from build123d import *

# Parameters (mm, degrees)
F1_DEPTH       = 10
F3_D           = 3.3
F3_CSINK_D     = 6
F3_CSINK_ANGLE = 90
F5_D           = 3.3
F5_CSINK_D     = 6
F5_CSINK_ANGLE = 90


with BuildPart() as f1:
    # F0 (on Front) → F1 (new body)
    with BuildSketch(Plane.XZ):
        Polygon((0, 44), (0, 0), (-15.65, -1.5), (-30.9, 0), (-30.9, 42), (-42.9, 42), (-42.9, 35), (-34.9, 35), (-34.9, -4), (-8, -4), (-8, -11), (4, -11), (4, 48), (-42.9, 48), (-42.9, 44), (-30.9, 44), (-15.65, 45.5), align=None)
    extrude(amount=F1_DEPTH)

    # F3 (through all)
    with Locations(Plane(origin=(0, 0, 35), x_dir=(1, 0, 0), z_dir=(0, 0, -1))):
        with Locations((-38.9, 5)):
            CounterSinkHole(F3_D / 2, F3_CSINK_D / 2, counter_sink_angle=F3_CSINK_ANGLE)

    # F5 (through all)
    with Locations(Plane(origin=(-8, 0, 0), x_dir=(0, -1, 0), z_dir=(-1, 0, 0))):
        with Locations((5, -7.5)):
            CounterSinkHole(F5_D / 2, F5_CSINK_D / 2, counter_sink_angle=F5_CSINK_ANGLE)


solid = f1.part
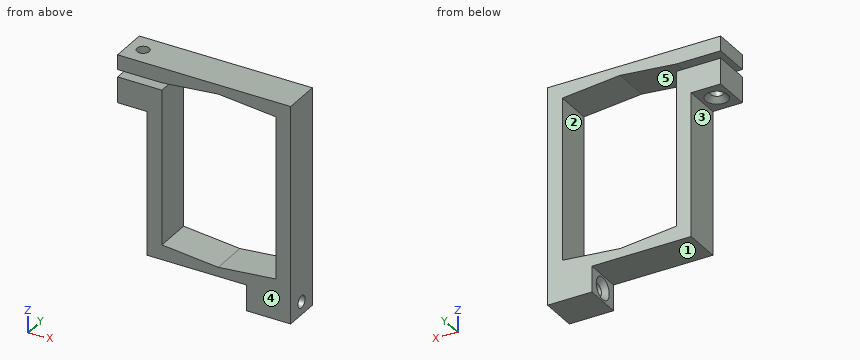
Can you work these out from the model? Positions are in its coordinate system, mm. Face numbers are marked on the shaded views. A direction names the side the tool comes from. Coordinates: 2 decimals unless noted, no trailing zeros. Order: outer loops, then holes, each group sorted by start corner. A loop starts at its lowest first (then second) coordinate and runs counter-clockwise, first axis right, second up. Notation, with made-up numbers: M -7,76 L 12,76 A10 cw 12,94 Z; hole C 7,42 d7. An arc over 180 degrees is marked long. Write item = value, one per line.
(1) Suppose I cut it at A-A on z = 27. Please give me the cut outline in (x, y).
Results are:
outline = M -34.9,-10 L -30.9,-10 L -30.9,0 L -34.9,0 Z; M 0,-10 L 4,-10 L 4,0 L 0,0 Z
(2) Suppose I cut it at C-C on x = -1.5. Please give me the cut outline in (y, z).
Results are:
outline = M -10,-11 L 0,-11 L 0,-0.14 L -10,-0.14 Z; M -10,44.14 L 0,44.14 L 0,48 L -10,48 Z; hole C -5,-7.5 d3.3
(3) Suppose I cut it at B-B on y = -5. State how many separate pieces and enclosed holes the cut face has, plus the area to 3 significant figures.
Results are:
separate_pieces = 4
enclosed_holes = 0
area = 701 mm2
(4) For pin 1 Ø3 at (y, z) = (-3, 28) entering from -X; pin 2 Ø3 at (x, y) = (-16.5, -4.5) entering from -Z; pin 3 Ø5.5 at (y, z) = (-3.5, -7.5) entering from -X; pin 4 Ø2.5 at (x, y) = (-38.9, -5) entering from +Z, each with a flat end and sliding along its axis, tell me the tip position at first contact or that it passes through.
Results are:
pin_1 = -34.9
pin_2 = -4
pin_3 = -8
pin_4 = through
(5) For the marked faces 4 and 5, which set-ups out of +Z, -Z, +X, -X, +Y, -Y let a thin tool reach every point of the face, with its end or its side?
Results are:
face_4 = +Z, -Z, +X, -X, -Y
face_5 = +Y, -Y
(6) Suppose I cut it at D-D on x = -21. Please give me the cut outline in (y, z).
Results are:
outline = M -10,-4 L 0,-4 L 0,-0.97 L -10,-0.97 Z; M -10,44.97 L 0,44.97 L 0,48 L -10,48 Z
(7) If we mould it in two halves opening along Z, with no side actions, what happens to the marked faces 1, 2 and 3? For each: pulls with the +Z half, pulls with the -Z half, needs draft (parallel to the pull), parting line crosses it, or undercut.
Results are:
face_1 = pulls with the -Z half
face_2 = undercut
face_3 = needs draft
(8) I need wall thicknesses on line 1 along X through (y, z) = (-5, 37.5); line 2 along X through (y, z) = (-8.5, 6.5); line 3 along Z through (x, y) = (-15.5, -7.5). Which ranges of each line are inside material? Lowest first, please. Write a range as [from, to].
Results are:
line_1 = [-42.9, -40.55], [-37.25, -30.9], [0, 4]
line_2 = [-34.9, -30.9], [0, 4]
line_3 = [-4, -1.49], [45.49, 48]
